The model under review builds one solid part; all positions refer to its coordinate system, in mm. Face numbers are marked on the shaded views. A direction names the side the tool comes from. Coordinates: 2 decimals unless noted, no trailing zeros. Order: outer loops, then holes, each group sorted by start corner. A loop starts at its lowest first (then second) coordinate and runs counter-clockwise, first axis right, second up. Notation, with made-up numbers: (75.25, 67) - (121.25, 67) arc R7 ccw to (121.25, 79) - close; hole circle Ø6 at (2.25, 24). An arc over 180 degrees is marked (long way). Answer in a Markdown table with one row per item.
```python
from build123d import *

# Parameters (mm, degrees)
SKETCH1_R          = 250
EXTRUDE1_DEPTH     = 300
SKETCH2_R          = 5
CUT_EXTRUDE1_DEPTH = 20
SKETCH3_R          = 200
SKETCH3_R_2        = 89.818842926
CUT_EXTRUDE2_DEPTH = 100
SKETCH4_R          = 89.818842926
CUT_EXTRUDE3_DEPTH = 20
FILLET1_R          = 10
SKETCH6_R          = 73.258337553
SKETCH6_R_2        = 63.258337553
CUT_EXTRUDE4_DEPTH = 10


with BuildPart() as part:
    # Sketch1 → Extrude1 (new body)
    with BuildSketch(Plane.XY):
        Circle(SKETCH1_R)
    extrude(amount=EXTRUDE1_DEPTH)

    # Sketch2 → Cut-Extrude1 (cut)
    with BuildSketch(Plane.XY.offset(300)):
        Circle(SKETCH2_R)
    extrude(amount=-CUT_EXTRUDE1_DEPTH, mode=Mode.SUBTRACT)

    # Sketch3 → Cut-Extrude2 (cut)
    with BuildSketch(Plane(origin=(0, 0, 0), x_dir=(-1, 0, 0), z_dir=(0, 0, -1))):
        Circle(SKETCH3_R)
        Circle(SKETCH3_R_2, mode=Mode.SUBTRACT)
    extrude(amount=-CUT_EXTRUDE2_DEPTH, mode=Mode.SUBTRACT)

    # Sketch4 → Cut-Extrude3 (cut)
    with BuildSketch(Plane(origin=(0, 0, 0), x_dir=(-1, 0, 0), z_dir=(0, 0, -1))):
        Circle(SKETCH4_R)
    extrude(amount=-CUT_EXTRUDE3_DEPTH, mode=Mode.SUBTRACT)

    # Sketch5 → Revolve1 (revolve)
    with BuildSketch(Plane(origin=(0, 0, 0), x_dir=(1, 0, 0), z_dir=(0, 1, 0))):
        with BuildLine():
            Line((0, -20), (0, 0))
            ThreePointArc((0, 0), (-46.360181472, -3.484720731), (-89.818842926, -20))
            Line((-89.818842926, -20), (0, -20))
        make_face()
    revolve(axis=Axis((0, 0, 20), (0, 0, -1)))

    # Fillet1
    fillet1_edges = [part.edges().sort_by_distance(p)[0] for p in [
        (-250, 0, 0),
        (-250, 0, 300),
    ]]
    fillet(fillet1_edges, radius=FILLET1_R)

    # Sketch6 → Cut-Extrude4 (cut)
    with BuildSketch(Plane.XY.offset(300)):
        Circle(SKETCH6_R)
        Circle(SKETCH6_R_2, mode=Mode.SUBTRACT)
    extrude(amount=-CUT_EXTRUDE4_DEPTH, mode=Mode.SUBTRACT)


solid = part.part
```
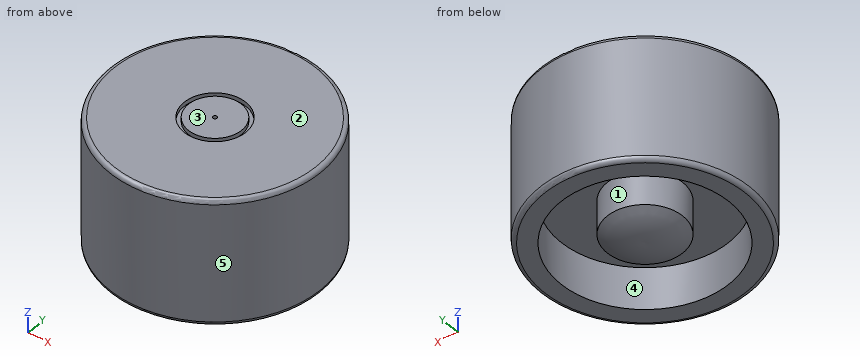
Item 1: To check wall thickness, follow line 1 (Y direction, x = 0, z = 295.75); line 2 (Y direction, x = 0, z = 294); line 3 (Y direction, x = 18, z = 84.5). State the ranges of each line that lie inside material, in increasing order. Write a range as from..to.
Check values:
| item | result |
|---|---|
| line 1 | -248.18..-73.26, -63.26..-5, 5..63.26, 73.26..248.18 |
| line 2 | -249.17..-73.26, -63.26..-5, 5..63.26, 73.26..249.17 |
| line 3 | -249.35..-199.19, -88..88, 199.19..249.35 |
Item 2: Mouldability with a two-part tool opening along Y and no side actions: class the marked faces 3, 4 and 5 as +Y half, -Y half, draft (parallel to the pull), parting line (faces both ways), or undercut.
Check values:
| item | result |
|---|---|
| face 3 | draft |
| face 4 | undercut |
| face 5 | parting line |
Item 3: We need section B-B, the plane z = 175. Write out the cut boundary in (x, y).
Check values:
| item | result |
|---|---|
| outline | circle Ø500 at (0, 0) |
Item 4: We need section A-A, the plane z = 39.5. Write out the cut boundary in (x, y).
Check values:
| item | result |
|---|---|
| outline | circle Ø500 at (0, 0); circle Ø179.64 at (0, 0); hole circle Ø400 at (0, 0) |
Item 5: Clearance check with flat-ended pins moving along their axes: pin 1 Ø6 at (y, z) = (-171, 38) entering from -X; pin 2 Ø12 at (x, y) = (2.5, -198) entering from -Z; pin 3 Ø10 at (x, y) = (-119.5, -81) entering from -Z. State where each tip first meets the part, or that it passes through.
Check values:
| item | result |
|---|---|
| pin 1 | x = -185.14 |
| pin 2 | z = 0 |
| pin 3 | z = 100 |
Item 6: Tool access review of the marked faces 1 and 2: name each direction out of +Z, -Z, +X, -X, +Y, -Y from which nothing blocks a thin tool from reaching the whole face with its end or side.
Check values:
| item | result |
|---|---|
| face 1 | -Z |
| face 2 | +Z, +X, -X, +Y, -Y |
